from build123d import *

# Parameters (mm, degrees)
SKETCH_1_R          = 13.5
EXTRUDE_1_DEPTH     = 8
SKETCH_3_W          = 45
SKETCH_3_H          = 12
EXTRUDE_2_DEPTH     = 8
SKETCH_2_R          = 4
CUT_EXTRUDE_1_DEPTH = 8
SKETCH_4_R          = 2.5
CUT_EXTRUDE_2_DEPTH = 9
FILLET_1_R          = 3


with BuildPart() as part:
    # 草图1 → 凸台-拉伸1 (new body)
    with BuildSketch(Plane.XY):
        Circle(SKETCH_1_R)
    extrude(amount=EXTRUDE_1_DEPTH)

    # 草图3 → 凸台-拉伸2 (add)
    with BuildSketch(Plane.XY.offset(8)):
        Rectangle(SKETCH_3_W, SKETCH_3_H)
    extrude(amount=-EXTRUDE_2_DEPTH)

    # 草图2 → 切除-拉伸1 (cut)
    with BuildSketch(Plane(origin=(0, 0, 0), x_dir=(-1, 0, 0), z_dir=(0, 0, -1))):
        Circle(SKETCH_2_R)
    extrude(amount=-CUT_EXTRUDE_1_DEPTH, mode=Mode.SUBTRACT)

    # 草图4 → 切除-拉伸2 (cut, through all)
    with BuildSketch(Plane(origin=(0, 0, 0), x_dir=(-1, 0, 0), z_dir=(0, 0, -1))):
        with Locations((-17.5, 0)):
            Circle(SKETCH_4_R)
        with Locations((17.5, 0)):
            Circle(SKETCH_4_R)
    extrude(amount=-CUT_EXTRUDE_2_DEPTH, mode=Mode.SUBTRACT)

    # 圆角1
    fillet_1_edges = [part.edges().sort_by_distance(p)[0] for p in [
        (-22.5, 6, 4),
        (22.5, -6, 4),
        (-22.5, -6, 4),
        (22.5, 6, 4),
    ]]
    fillet(fillet_1_edges, radius=FILLET_1_R)


solid = part.part
Can you work these out from the model? Positions are in its coordinate system, mm. A direction names the side the tool comes from. Coordinates: 2 decimals unless noted, no trailing zeros. Order: outer loops, then holes, each group sorted by start corner. A loop starts at its lowest first (then second) coordinate and runs counter-clockwise, first axis right, second up. Notation, with made-up numbers: M -38.75,27.5 L -20.75,27.5 A24 cw -20.75,41.5 Z; hole C 63,23.5 d10. An arc over 180 degrees is marked long. Write item = value, one per line.
(1) I need wall thicknesses on line 1 along Y through (x, z) = (0, 6.25); line 2 along X through (y, z) = (-1, 5); line 3 along Y through (x, z) = (17.5, 3.5). Which ranges of each line are inside material? Lowest first, please. Write a range as [from, to].
Results are:
line_1 = [-13.5, -4], [4, 13.5]
line_2 = [-22.5, -19.79], [-15.21, -3.87], [3.87, 15.21], [19.79, 22.5]
line_3 = [-6, -2.5], [2.5, 6]
(2) Suppose I cut it at C-C on z = 7.5. Please give me the cut outline in (x, y).
Results are:
outline = M -22.5,-3 A3 ccw -19.5,-6 L -12.09,-6 A13.5 ccw 12.09,-6 L 19.5,-6 A3 ccw 22.5,-3 L 22.5,3 A3 ccw 19.5,6 L 12.09,6 A13.5 ccw -12.09,6 L -19.5,6 A3 ccw -22.5,3 Z; hole C -17.5,0 d5; hole C 0,0 d8; hole C 17.5,0 d5
(3) For pin 1 Ø4.5 at (x, y) = (-17.5, 0) entering from -Z; pin 2 Ø2 at (x, z) = (-15.5, 5.5) entering from -Y; pin 3 Ø3.5 at (x, z) = (15.5, 5) entering from +Y; pin 4 Ø1 at (y, z) = (5, 2) entering from +X, each with a flat end and sliding along its axis, tell me the tip position at first contact or that it passes through.
Results are:
pin_1 = through
pin_2 = -6
pin_3 = 6
pin_4 = 22.1
(4) Suppose I cut it at B-B on y = 0. Please give me the cut outline in (x, z).
Results are:
outline = M -22.5,0 L -20,0 L -20,8 L -22.5,8 Z; M -15,0 L -4,0 L -4,8 L -15,8 Z; M 4,0 L 15,0 L 15,8 L 4,8 Z; M 20,0 L 22.5,0 L 22.5,8 L 20,8 Z
(5) For faces 4 (the face through (-16, 6, 4)), 5 (the face through (16, -6, 4)), 6 (the face through (16, 6, 4)), which set-ups out of +Z, -Z, +X, -X, +Y, -Y let a thin tool reach every point of the face, with its end or its side?
Results are:
face_4 = +Z, -Z, -X, +Y
face_5 = +Z, -Z, +X, -Y
face_6 = +Z, -Z, +X, +Y
(6) Suppose I cut it at D-D on y = 9.5. Please give me the cut outline in (x, z), plus the area to 3 significant figures.
Results are:
outline = M -9.59,0 L 9.59,0 L 9.59,8 L -9.59,8 Z
area = 153 mm2
(7) Suppose I cut it at A-A on x = 17.5. Please give me the cut outline in (y, z), plus the area to 3 significant figures.
Results are:
outline = M -6,0 L -2.5,0 L -2.5,8 L -6,8 Z; M 2.5,0 L 6,0 L 6,8 L 2.5,8 Z
area = 56.0 mm2
(8) If we mould it in two halves opening along Y, with no side actions, what happens to faces 1 (the face through (5, 0, 0)), 2 (the face through (-15, 0, 4)), 3 (the face through (21.6, 5.14, 3.94))? For each: pulls with the +Y half, pulls with the -Y half, needs draft (parallel to the pull), parting line crosses it, or undercut.
Results are:
face_1 = needs draft
face_2 = undercut
face_3 = pulls with the +Y half
